Part model, mm, in its own coordinate system. A direction names the side the tool comes from. Give positions to 0.01 mm unless a question says otherwise; leave off trailing zeros. Order: outer loops, then holes, each group sorted by start corner. A loop starts at its lowest first (then second) coordinate and runs counter-clockwise, first axis right, second up.
1. Slice it at B-B on x = 5. List the corners of the cut face in (y, z) (3 decimals), and give its area (3 significant figures).
2. Probe line 1 (Z direction, x = 9.5, y = 13.25); line 2 (Z direction, x = 9, y = 13.75); line 3 (Z direction, x = 12, y = 3). List the from-to ranges inside material, lowest first.
3. Slice it at D-D on z = -7.75. List the corners of the cut face in (x, y) (3 decimals).
4. Drop flat-ended pins along their axis: pin 1 Ø1 at (x, y) = (8, 13.5) entering from +Z; pin 2 Ø6 at (x, z) = (9.5, -9) entering from +Y (3 decimals); pin 3 Ø3 at (x, y) = (11, 5) entering from -Z; pin 4 Ø5 at (x, y) = (3.175, 9.525) entering from -Z (3 decimals). Give the stop position or say it passes through.
5. Slice it at A-A on y = 5. List the corners of the cut face in (x, z) (3 decimals), and give its area (3 significant figures).
6. Slice it at C-C on z = -13.5. List the corners of the cut face in (x, y) (3 decimals).
7. Mould opens along Z. For faces 1 (the flat face through (9, 3.175, -10)), 2 (the flat face through (12.7, 8, -13)), 3 (the flat face through (9, 8, -19.05)) say: +Z half, -Z half, draft (parallel to the pull), parting line (faces both ways), or undercut.
8. Which spindle directions (+Z, -Z, +X, -X, +Y, -Y) get a long thin tool onto all of the face, cutting with end or side? Do faces 4 (the flat face through (3.175, 3, -3)), 5 (the flat face through (6.35, 6, -21)), 6 (the flat face through (9, 14, -6.35)), 7 (the cylindrical face through (6.88, 9.61, -9.64)), 8 (the cylindrical face through (0.65, 3.97, -15.96)). Say none if no direction does.
from build123d import *

# Parameters (mm, degrees)
SKETCH1_W                = 6.35
SKETCH1_H                = 15.875
SKETCH1_W_2              = 15.875
SKETCH1_H_2              = 6.35
BOSS_EXTRUDE1_DEPTH      = 6.35
SKETCH5_R                = 2.645833291
CUT_EXTRUDE1_DEPTH       = 12.7
SKETCH6_R                = 2.645833333
CUT_EXTRUDE2_DEPTH       = 12.7
SKETCH10_W               = 6.35
SKETCH10_H               = 15.875
BOSS_EXTRUDE5_DEPTH      = 6.35
SKETCH11_R               = 2.645833333
CUT_EXTRUDE5_DEPTH       = 12.7
SKETCH12_R               = 2.645833333
CUT_EXTRUDE6_DEPTH       = 12.7
SKETCH13_W               = 6.35
SKETCH13_H               = 12.7
BOSS_EXTRUDE6_DEPTH      = 3.175
BOSS_EXTRUDE6_DEPTH_BACK = 12.7
SKETCH14_R               = 2.645833333
CUT_EXTRUDE7_DEPTH       = 12.7


with BuildPart() as part:
    # Sketch1 → Boss-Extrude1 (new body)
    with BuildSketch(Plane(origin=(0, 0, 0), x_dir=(1, 0, 0), z_dir=(0, 1, 0))):
        with Locations((3.175, 14.2875)):
            Rectangle(SKETCH1_W, SKETCH1_H)
        with Locations((7.9375, 3.175)):
            Rectangle(SKETCH1_W_2, SKETCH1_H_2)
    extrude(amount=BOSS_EXTRUDE1_DEPTH)

    # Sketch5 → Cut-Extrude1 (cut)
    with BuildSketch(Plane(origin=(15.875, 0, 0), x_dir=(0, 0, -1), z_dir=(1, 0, 0))):
        with Locations((3.175, 3.175)):
            Circle(SKETCH5_R)
    extrude(amount=-CUT_EXTRUDE1_DEPTH, mode=Mode.SUBTRACT)

    # Sketch6 → Cut-Extrude2 (cut)
    with BuildSketch(Plane(origin=(0, 0, -22.225), x_dir=(-1, 0, 0), z_dir=(0, 0, -1))):
        with Locations((-3.175, 3.175)):
            Circle(SKETCH6_R)
    extrude(amount=-CUT_EXTRUDE2_DEPTH, mode=Mode.SUBTRACT)

    # Sketch10 → Boss-Extrude5 (add)
    with BuildSketch(Plane(origin=(0, 6.35, 0), x_dir=(1, 0, 0), z_dir=(0, 1, 0))):
        with Locations((3.175, 14.2875)):
            Rectangle(SKETCH10_W, SKETCH10_H)
        Polygon((0, 6.35), (0, 0), (15.875, 0), (15.875, 6.35), (6.35, 6.35), align=None)
    extrude(amount=BOSS_EXTRUDE5_DEPTH)

    # Sketch11 → Cut-Extrude5 (cut)
    with BuildSketch(Plane(origin=(15.875, 0, 0), x_dir=(0, 0, -1), z_dir=(1, 0, 0))):
        with Locations((3.175, 9.525)):
            Circle(SKETCH11_R)
    extrude(amount=-CUT_EXTRUDE5_DEPTH, mode=Mode.SUBTRACT)

    # Sketch12 → Cut-Extrude6 (cut)
    with BuildSketch(Plane(origin=(0, 0, -22.225), x_dir=(-1, 0, 0), z_dir=(0, 0, -1))):
        with Locations((-3.175, 9.525)):
            Circle(SKETCH12_R)
    extrude(amount=-CUT_EXTRUDE6_DEPTH, mode=Mode.SUBTRACT)

    # Sketch13 → Boss-Extrude6 (add, two sides)
    with BuildSketch(Plane(origin=(0, 12.7, 0), x_dir=(1, 0, 0), z_dir=(0, 1, 0))) as boss_extrude6_sk:
        with Locations((9.525, 12.7)):
            Rectangle(SKETCH13_W, SKETCH13_H)
    extrude(amount=BOSS_EXTRUDE6_DEPTH)
    extrude(boss_extrude6_sk.sketch, amount=-BOSS_EXTRUDE6_DEPTH_BACK)

    # Sketch14 → Cut-Extrude7 (cut)
    with BuildSketch(Plane(origin=(0, 15.875, 0), x_dir=(1, 0, 0), z_dir=(0, 1, 0))):
        with Locations((9.525, 9.525)):
            Circle(SKETCH14_R)
        with Locations((9.525, 15.875)):
            Circle(SKETCH14_R)
    extrude(amount=-CUT_EXTRUDE7_DEPTH, mode=Mode.SUBTRACT)


solid = part.part
Data:
1. outline: (0, -22.225) - (1.259, -22.225) - (1.259, -9.525) - (5.091, -9.525) - (5.091, -22.225) - (7.609, -22.225) - (7.609, -9.525) - (11.441, -9.525) - (11.441, -22.225) - (12.7, -22.225) - (12.7, 0) - (0, 0) - close; hole circle Ø5.292 at (3.175, -3.175); hole circle Ø5.292 at (9.525, -3.175)
1. area: 141 mm2
2. line 1: z = -19.05 to -18.52, -13.23 to -12.17, -6.88 to -6.35
2. line 2: z = -19.05 to -18.47, -13.28 to -12.12, -6.93 to -6.35
2. line 3: z = -19.05 to -5.82, -0.53 to 0
3. outline: (0, 0) - (12.7, 0) - (12.7, 15.875) - (11.487, 15.875) - (11.487, 3.175) - (7.563, 3.175) - (7.563, 15.875) - (6.35, 15.875) - (6.35, 12.7) - (0, 12.7) - close
4. pin 1: stops at z = -6.35
4. pin 2: stops at y = 15.875
4. pin 3: stops at z = -19.05
4. pin 4: stops at z = -9.525
5. outline: (0, -22.225) - (1.259, -22.225) - (1.259, -9.525) - (5.091, -9.525) - (5.091, -22.225) - (6.35, -22.225) - (6.35, -19.05) - (12.7, -19.05) - (12.7, -6.35) - (15.875, -6.35) - (15.875, -5.091) - (3.175, -5.091) - (3.175, -1.259) - (15.875, -1.259) - (15.875, 0) - (0, 0) - close; hole circle Ø5.292 at (9.525, -15.875); hole circle Ø5.292 at (9.525, -9.525)
5. area: 141 mm2
6. outline: (0, 0) - (12.7, 0) - (12.7, 15.875) - (10.691, 15.875) - (10.691, 3.175) - (8.359, 3.175) - (8.359, 15.875) - (6.35, 15.875) - (6.35, 12.7) - (0, 12.7) - close; hole circle Ø5.292 at (3.175, 3.175); hole circle Ø5.292 at (3.175, 9.525)
7. face 1: undercut
7. face 2: draft
7. face 3: -Z half
8. face 4: +X
8. face 5: -Z, +X, +Y, -Y
8. face 6: +Z, +X, -X, +Y
8. face 7: +Y
8. face 8: -Z
